```python
from build123d import *

# Parameters (mm, degrees)
EXTRUDE_1_DEPTH               = 38
SKETCH_2_W                    = 52
SKETCH_2_H                    = 26
CUT_EXTRUDE_1_DEPTH           = 273.053680503
EXTRUDE_2_DEPTH               = 26
HOLE_WIZARD_M36_1_D           = 38
HOLE_WIZARD_M36_1_CBORE_D     = 57
HOLE_WIZARD_M36_1_CBORE_DEPTH = 1
FILLET_2_R                    = 6


with BuildPart() as part:
    # 스케치1 → 보스-돌출1 (new, symmetric)
    with BuildSketch(Plane.XY):
        Polygon((0, 0), (127, 0), (127, 50), (38, 139), (0, 139), align=None)
    extrude(amount=EXTRUDE_1_DEPTH, both=True)

    # 스케치2 → 컷-돌출1 (cut, through all, along a direction that is not the sketch's normal)
    with BuildSketch(Plane(origin=(0, 139, 0), x_dir=(1, 0, 0), z_dir=(0, 1, 0))):
        with Locations((38, 0)):
            Rectangle(SKETCH_2_W, SKETCH_2_H)
    extrude(amount=-CUT_EXTRUDE_1_DEPTH, dir=(-0.7071067811865512, 0.7071067811865438, 0), mode=Mode.SUBTRACT)

    # 스케치3 → 보스-돌출2 (add)
    with BuildSketch(Plane.XZ):
        with BuildLine():
            Line((6, 38), (82, 38))
            Line((82, 38), (82, 89))
            ThreePointArc((82, 89), (44, 127), (6, 89))
            Line((6, 89), (6, 38))
        make_face()
    extrude_2 = extrude(amount=-EXTRUDE_2_DEPTH)

    # M36 소켓 머리 캡 나사용 카운터보어1 (through all)
    with Locations(Plane(origin=(0, 26, 0), x_dir=(1, 0, 0), z_dir=(0, 1, 0))):
        with Locations((44, -89)):
            hole_wizard_m36_1 = CounterBoreHole(HOLE_WIZARD_M36_1_D / 2, HOLE_WIZARD_M36_1_CBORE_D / 2, HOLE_WIZARD_M36_1_CBORE_DEPTH)

    # 대칭 복사1: 보스-돌출2, M36 소켓 머리 캡 나사용 카운터보어1 across plane
    add(extrude_2.mirror(Plane.XY))
    add(hole_wizard_m36_1.mirror(Plane.XY), mode=Mode.SUBTRACT)

    # 필렛2
    fillet_2_edges = [part.edges().sort_by_distance(p)[0] for p in [
        (6, 26, 63.5),
        (6, 13, 38),
        (44, 26, 127),
        (82, 26, 63.5),
        (44, 26, 38),
        (82, 13, 38),
        (6, 13, -38),
        (82, 13, -38),
        (6, 26, -63.5),
        (44, 26, -38),
        (82, 26, -63.5),
        (44, 26, -127),
    ]]
    fillet(fillet_2_edges, radius=FILLET_2_R - 0.0001)  # a hair under: the kernel refuses the full size


solid = part.part
```
Here's how the part is built. I have some questions about the finished solid (model axes, mm). A direction names the side the tool comes from. Give positions to 0.01 mm unless a question says otherwise; leave off trailing zeros. Order: outer loops, then holes, each group sorted by start corner. A loop starts at its lowest first (then second) coordinate and runs counter-clockwise, first axis right, second up. Notation, with made-up numbers: (8, -21.5) - (51, -21.5) arc R23 cw to (51, -6.5) - close; hole circle Ø11 at (68.5, 53.5). An arc over 180 degrees is marked (long way). Answer as a JSON object with one key per item and string values. Group by question number.
Item 1: Which directions (+Z, -Z, +X, -X, +Y, -Y) give clear straight access to the entire face, cutting with the end or side of a thin tool? Please do faces 5 (the flat face through (6, 10, -67)), 6 (the flat face through (78, 90, 13)), 7 (the flat face through (82, 10, 66)), 8 (the cylindrical face through (57.151, 25.507, 114.284)).
Item 2: Please list where these lines run through material, in increasing order: probe 1 along Z at (x, y) = (44, 18); probe 2 along X at (y, z) = (9, -89); probe 3 along Z at (x, y) = (77, 82).
Item 3: If we mould it in two halves opening along X, with no side actions, what happens to faces 1 (the cylindrical face through (46.47, 12.32, 70.16)), 2 (the cylindrical face through (7.711, 24.196, 66.185)), 3 (the flat face through (83, 94, -25)), 4 (the flat face through (78, 90, -13))? For each: pulls with the +X half, pulls with the -X half, needs draft (parallel to the pull), parting line crosses it, or undercut.
Item 4: If we section it at A-A on x = 44: Give the number of separate pieces and of enclosed holes in the cut face, and give its area (3 significant figures).
Item 5: If we section it at D-D on x = 118.5: Please give me the cut outline in (y, z), and give its area (3 significant figures).
Item 6: For P1, Ø5, axis at x = 13.5, y = 83.5, coming from the +Z side; P2, Ø12, axis at y = 60.5, z = 29.5, coming from the +X side; P3, Ø10, axis at x = 44, y = 46.5, coming from the -Z side; P4, Ø1, axis at x = 14.5, z = 32.5, coming from the -Y side, each with a flat end and sliding along its axis, tell me the tip position at first contact or that it passes through.
Item 7: If we section it at C-C on z = -80: Please give me the cut outline in (x, y), and give its area (3 significant figures).
Result set:
{
 "1": {"face 5": "-Z, -X, +Y, -Y", "face 6": "+X, +Y", "face 7": "+Z, +X, +Y, -Y", "face 8": "+Y"},
 "2": {"probe 1": "-127 to -108, -70 to 70, 108 to 127", "probe 2": "6 to 25, 63 to 82", "probe 3": "-38 to -13, 13 to 38"},
 "3": {"face 1": "undercut", "face 2": "pulls with the -X half", "face 3": "pulls with the +X half", "face 4": "needs draft"},
 "4": {"separate pieces": "3", "enclosed holes": "0", "area": "12,000 mm²"},
 "5": {"outline": "(0, -38) - (58.5, -38) - (58.5, -13) - (32.5, -13) - (32.5, 13) - (58.5, 13) - (58.5, 38) - (0, 38) - close", "area": "3,770 mm²"},
 "6": {"P1": "z = 38", "P2": "x = 122.5", "P3": "z = -38", "P4": "y = 0"},
 "7": {"outline": "(6, 0) - (27.27, 0) - (27.27, 25) - (16.96, 25) - (16.96, 26) - (12, 26) arc R6 ccw to (6, 20) - close; (60.73, 0) - (82, 0) - (82, 20) arc R6 ccw to (76, 26) - (71.04, 26) - (71.04, 25) - (60.73, 25) - close", "area": "1,070 mm²"}
}
